```python
from build123d import *

# Parameters (mm, degrees)
SKETCH1_R           = 17.435
BOSS_EXTRUDE2_DEPTH = 558.8
CHAMFER2_SIZE       = 6
CHAMFER2_SIZE2      = 3.464101615
CHAMFER3_SIZE       = 3.5
CHAMFER3_SIZE2      = 2.020725942
CUT_EXTRUDE1_DEPTH  = 558.8


with BuildPart() as part:
    # Sketch1 → Boss-Extrude2 (new body)
    with BuildSketch(Plane.XY):
        Circle(SKETCH1_R)
    extrude(amount=BOSS_EXTRUDE2_DEPTH)

    # Chamfer2
    chamfer2_edges = [part.edges().sort_by_distance(p)[0] for p in [
        (-17.435, 0, 558.8),
    ]]
    chamfer2_side = [part.faces().sort_by_distance(p)[0] for p in [
        (-17.435, 0, 279.4),
    ]]
    chamfer(chamfer2_edges, length=CHAMFER2_SIZE, length2=CHAMFER2_SIZE2, reference=chamfer2_side[0])

    # Chamfer3
    chamfer3_edges = [part.edges().sort_by_distance(p)[0] for p in [
        (-17.435, 0, 0),
    ]]
    chamfer3_side = [part.faces().sort_by_distance(p)[0] for p in [
        (0, 0, 0),
    ]]
    chamfer(chamfer3_edges, length=CHAMFER3_SIZE, length2=CHAMFER3_SIZE2, reference=chamfer3_side[0])

    # Sketch3 → Cut-Extrude1 (cut)
    with BuildSketch(Plane(origin=(0, 0, 0), x_dir=(-1, 0, 0), z_dir=(0, 0, -1))):
        with BuildLine():
            Line((-4.32, 16.891323956), (-4.32, 13.258982804))
            ThreePointArc((-4.32, 13.258982804), (-6.9725, 12.076724256), (-9.322615937, 10.370721146))
            Line((-9.322615937, 10.370721146), (-12.46831565, 12.186891723))
            ThreePointArc((-12.46831565, 12.186891723), (-8.7175, 15.099152915), (-4.32, 16.891323956))
        make_face()
        with BuildLine():
            Line((12.46831565, 12.186891723), (9.322615937, 10.370721146))
            ThreePointArc((9.322615937, 10.370721146), (6.9725, 12.076724256), (4.32, 13.258982804))
            Line((4.32, 13.258982804), (4.32, 16.891323956))
            ThreePointArc((4.32, 16.891323956), (8.7175, 15.099152915), (12.46831565, 12.186891723))
        make_face()
        with BuildLine():
            Line((16.78831565, 4.704432234), (13.642615937, 2.888261658))
            ThreePointArc((13.642615937, 2.888261658), (13.945, 0), (13.642615937, -2.888261658))
            Line((13.642615937, -2.888261658), (16.78831565, -4.704432234))
            ThreePointArc((16.78831565, -4.704432234), (17.435, 0), (16.78831565, 4.704432234))
        make_face()
        with BuildLine():
            Line((12.46831565, -12.186891723), (9.322615937, -10.370721146))
            ThreePointArc((9.322615937, -10.370721146), (6.9725, -12.076724256), (4.32, -13.258982804))
            Line((4.32, -13.258982804), (4.32, -16.891323956))
            ThreePointArc((4.32, -16.891323956), (8.7175, -15.099152915), (12.46831565, -12.186891723))
        make_face()
        with BuildLine():
            Line((-4.32, -16.891323956), (-4.32, -13.258982804))
            ThreePointArc((-4.32, -13.258982804), (-6.9725, -12.076724256), (-9.322615937, -10.370721146))
            Line((-9.322615937, -10.370721146), (-12.46831565, -12.186891723))
            ThreePointArc((-12.46831565, -12.186891723), (-8.7175, -15.099152915), (-4.32, -16.891323956))
        make_face()
        with BuildLine():
            Line((-16.78831565, -4.704432234), (-13.642615937, -2.888261658))
            ThreePointArc((-13.642615937, -2.888261658), (-13.945, 0), (-13.642615937, 2.888261658))
            Line((-13.642615937, 2.888261658), (-16.78831565, 4.704432234))
            ThreePointArc((-16.78831565, 4.704432234), (-17.435, 0), (-16.78831565, -4.704432234))
        make_face()
    extrude(amount=-CUT_EXTRUDE1_DEPTH, mode=Mode.SUBTRACT)


solid = part.part
```
Build history of the part. All positions in model axes, mm. Give positions to 0.01 mm unless a question says otherwise; leave off trailing zeros. Loops run counter-clockwise (first coordinate to the right, second up) from the corner with the lowest first, then second, coordinate; pieces in that order, holes last.
Item 1: Flat gauge pins, fed straight in: pin 1 (1.5 mm diameter, centred on x = 8, z = 348, fed in from -Y); pin 2 (3 mm diameter, centred on x = -4.5, z = 183.5, fed in from +Y); pin 3 (8 mm diameter, centred on x = 7.5, z = 322.5, fed in from +Y). Where does each tip first touch, or does it go through?
Answers follow:
pin 1: stops at y = -11.91
pin 2: stops at y = 17.17
pin 3: stops at y = 17.08
Item 2: Drill centre lines: line 1 (X direction, y = 12, z = 306.5); line 2 (X direction, y = -11.5, z = 119); line 3 (Y direction, x = 1, z = 275.5). Where is each one in solid material? Low to high.
Answers follow:
line 1: x = -12.65 to -12.14, -7.1 to 7.1, 12.14 to 12.65
line 2: x = -13.1 to -11.28, -7.89 to 7.89, 11.28 to 13.1
line 3: y = -17.41 to 17.41
Item 3: Slice it at A-A, the plane z = 271. List the corners of the cut face in (x, y) (3 decimals), and give its area (3 significant figures).
Answers follow:
outline: (-16.788, -4.704) arc R17.435 ccw to (-12.468, -12.187) - (-9.323, -10.371) arc R13.945 ccw to (-4.32, -13.259) - (-4.32, -16.891) arc R17.435 ccw to (4.32, -16.891) - (4.32, -13.259) arc R13.945 ccw to (9.323, -10.371) - (12.468, -12.187) arc R17.435 ccw to (16.788, -4.704) - (13.643, -2.888) arc R13.945 ccw to (13.643, 2.888) - (16.788, 4.704) arc R17.435 ccw to (12.468, 12.187) - (9.323, 10.371) arc R13.945 ccw to (4.32, 13.259) - (4.32, 16.891) arc R17.435 ccw to (-4.32, 16.891) - (-4.32, 13.259) arc R13.945 ccw to (-9.323, 10.371) - (-12.468, 12.187) arc R17.435 ccw to (-16.788, 4.704) - (-13.643, 2.888) arc R13.945 ccw to (-13.643, -2.888) - close
area: 794 mm2
